Solid Edge part; units mm, degrees
sketch "Sketch1" plane through (0, 0, 0) normal (0, 0, 1) x (1, 0, 0)
  line L0 (-10, -10) -> (10, -10)
  line L1 (10, -10) -> (10, 10)
  line L2 (10, 10) -> (-10, 10)
  line L3 (-10, 10) -> (-10, 2.65)
  line L4 (-8.5, 2.65) -> (-10, 2.65)
  line L5 (-8.5, 4.25) -> (-8.5, 2.65)
  line L6 (-3.3, 4.25) -> (-8.5, 4.25)
  arc A0 (-3.3, 4.25) -> (-3.3, -4.25) centre (-8.5833, 0) cw
  line L7 (-8.5, -4.25) -> (-3.3, -4.25)
  line L8 (-8.5, -2.65) -> (-8.5, -4.25)
  line L9 (-10, -2.65) -> (-8.5, -2.65)
  line L10 (-10, -2.65) -> (-10, -10)
extrude "Protrusion1" add sketch "Sketch1" along normal blind 50
sketch "Sketch2" plane through (0, 10, 25) normal (0, 1, 0) x (0, 0, -1)
  line L0 (-25, -10) -> (-20, -10)
  line L1 (-20, -10) -> (-20, 10)
  line L2 (-20, 10) -> (-25, 10)
  line L3 (-25, 10) -> (-25, -10)
  line L4 (25, 10) -> (20, 10)
  line L5 (20, 10) -> (20, -10)
  line L6 (20, -10) -> (25, -10)
  line L7 (25, -10) -> (25, 10)
extrude "Protrusion2" add sketch "Sketch2" along normal blind 30
sketch "Sketch3" plane through (0, 15, 50) normal (0, 0, 1) x (0, 1, 0)
  arc A0 (15, -3) -> (17.5, -0.5) centre (15, -0.5) ccw
  line L0 (17.5, -0.5) -> (17.5, 0.5)
  arc A1 (17.5, 0.5) -> (15, 3) centre (15, 0.5) ccw
  line L1 (15, 3) -> (5, 3)
  arc A2 (5, 3) -> (2.5, 0.5) centre (5, 0.5) ccw
  line L2 (2.5, 0.5) -> (2.5, -0.5)
  arc A3 (5, -3) -> (2.5, -0.5) centre (5, -0.5) cw
  line L3 (5, -3) -> (15, -3)
extrude "Cutout1" cut sketch "Sketch3" against normal blind 70
Geometry check sheet. Reference: the model listing, model coordinates, mm. A direction names the side the tool comes from. Give positions to 0.01 mm unless a question says otherwise; leave off trailing zeros. Loops run counter-clockwise (first coordinate to the right, second up) from the corner with the lowest first, then second, coordinate; pieces in that order, holes last. Notation, with made-up numbers: M -5.5,-25 L 9.5,-25 A29 cw 9.5,13 Z; hole C 42,78.25 d4. An arc over 180 degrees is marked long. Write each question's results on one line, items separated by ' | '.
1) Section check D-D, the plane x = 1.25. Record the boundary of the cut face in (y, z), plus the area to 3 significant figures.
Answers follow:
outline: M -10,0 L 17.62,0 L 17.62,5 L 10,5 L 10,45 L 17.62,45 L 17.62,50 L -10,50 Z; M 32.38,0 L 40,0 L 40,5 L 32.38,5 Z; M 32.38,45 L 40,45 L 40,50 L 32.38,50 Z | area: 1,150 mm2
2) Section check B-B, the plane y = 34.5. Record the boundary of the cut face in (x, z).
Answers follow:
outline: M -10,0 L 10,0 L 10,5 L -10,5 Z; M -10,45 L 10,45 L 10,50 L -10,50 Z
3) Release check for a two-part mould opening along X. For faces 4 (the face through (-9, -2.65, 25)), 5 (the face through (-10, 9, 25)), 6 (the face through (-6, -4.25, 25)) record: +X half, -X half, draft (parallel to the pull), parting line (faces both ways), or undercut.
Answers follow:
face 4: draft | face 5: -X half | face 6: undercut
4) Section check A-A, the plane x = -7. Record the boundary of the cut face in (y, z), plus the area to 3 significant figures.
Answers follow:
outline: M -10,0 L -4.25,0 L -4.25,50 L -10,50 Z; M 4.25,0 L 40,0 L 40,5 L 10,5 L 10,45 L 40,45 L 40,50 L 4.25,50 Z | area: 875 mm2
5) Section check C-C, the plane y = 28. Record the boundary of the cut face in (x, z), plus the area to 3 significant figures.
Answers follow:
outline: M -10,0 L -3,0 L -3,5 L -10,5 Z; M -10,45 L -3,45 L -3,50 L -10,50 Z; M 3,0 L 10,0 L 10,5 L 3,5 Z; M 3,45 L 10,45 L 10,50 L 3,50 Z | area: 140 mm2
6) Gauge pin test, flat end, axial feed: pin 1 (5.5 mm diameter, centred on x = -4.5, z = 33.5, fed in from +Y). Record the tip position at first contact, or that the pin passes through.
Answers follow:
pin 1: y = 10
7) Tool access check on faces 1 (the face through (-3, 25, 48)), 2 (the face through (5, 25, 45)), 3 (the face through (10, 4, 25)). Record the directions out of +Z, -Z, +X, -X, +Y, -Y that give a thin tool (end or side, any length) a straight path to the whole face; none if there is none.
Answers follow:
face 1: +Z, -Z | face 2: +X, -X, +Y | face 3: +Z, -Z, +X, +Y, -Y
8) Thickness scan on line 1 (Z direction, x = 5, y = 31); line 2 (Y direction, x = -5.5, z = 11.5); line 3 (Y direction, x = -0.25, z = 37.5). Record the ranges inside material, lowest first.
Answers follow:
line 1: 0 to 5, 45 to 50 | line 2: -10 to -4.25, 4.25 to 10 | line 3: -10 to 10
